Could you check a few things on this model? Use its own coordinates, in mm. A direction names the side the tool comes from. Round coordinates to 2 decimals unless told otherwise and drop trailing zeros. Write each loop counter-clockwise with the first axis right and the second up, starting at its lowest first coordinate (ties: lowest second). Pieces come first, ordered by that corner, then holes. Notation, with made-up numbers: (-2, -39) -> (53, -39) arc R25 ccw to (53, -18) -> close; hole circle Ø2 at (-14, 23.25). An arc over 180 degrees is marked (long way). Answer as CSV lines item,"result". Start each with the question number.
Q1. For faces 1 (the flat face through (34.546, 29, -2)), 2 (the flat face through (26, 31.5, 0)), 3 (the cylindrical face through (22.627, 26.43, -0.488)), 4 (the flat face through (26.946, 0.74, -11.463)), 5 (the flat face through (35, 29, -4.224)), which set-ups out of +Z, -Z, +X, -X, +Y, -Y let a thin tool reach every point of the face, with its end or its side?
Q2. Imagine slicing it at B-B on z = 0.5. Please give me the cut outline in (x, y).
Q3. Imagine slicing it at A-A on y = 28.5. Please give me the cut outline in (x, z), and give its area (3 significant figures).
Q4. Will these pins go through, and if not, where does the flat tip stop? pin 1 Ø2 at (x, z) = (26, -6.5) entering from +Y; pin 2 Ø5 at (x, y) = (20, 5.5) entering from +Z; pin 3 Ø1 at (x, y) = (34.5, 28.5) entering from +Z (3 decimals).
Q5. Imagine slicing it at D-D on y = 12.5. Please give me the cut outline in (x, z), and give its area (3 significant figures).
Q6. If I drill on line 1 (Z direction, x = 26.25, y = 23.5); line 2 (Y direction, x = 33.5, z = 1); line 3 (X direction, y = 19.5, z = 5.75), over which ranges is the centre line in solid material (lowest first)? Write a range as [from, to].
Q7. Imagine slicing it at C-C on x = 25.25. Please give me the cut outline in (y, z), and give its area (3 significant figures).
Q8. If we mould it in two halves opening along Z, with no side actions, what happens to faces 6 (the flat face through (20.605, 28.895, 6.235)), 7 (the flat face through (37.85, 0.74, -0.616)), 8 (the cylindrical face through (30.467, 28.895, 7.089)), 9 (the flat face through (34, 1.5, -7))? For each: pulls with the +Z half, pulls with the -Z half, needs draft (parallel to the pull), parting line crosses it, or undercut.
from build123d import *

# Parameters (mm, degrees)
SKETCH1_R           = 10
SKETCH1_R_2         = 7.636363636
BOSS_EXTRUDE1_DEPTH = 21.5
BOSS_EXTRUDE2_DEPTH = 15
SKETCH3_R           = 3.75
BOSS_EXTRUDE3_DEPTH = 10
BOSS_EXTRUDE4_DEPTH = 1.5
SKETCH6_W           = 32.555421104
SKETCH6_H           = 30.593451785
BOSS_EXTRUDE5_DEPTH = 1.5
SKETCH8_W           = 32.555421103
SKETCH8_H           = 30.593451785
CUT_EXTRUDE1_DEPTH  = 1.5


# Read off the part's stored shape, not the designer's step: Boss-Extrude4
with BuildPart() as part:
    # Sketch1 → Boss-Extrude1 (new body)
    # profile 1 of 2: a face of its own
    with BuildSketch(Plane(origin=(0, 0, 0), x_dir=(1, 0, 0), z_dir=(0, 1, 0))):
        with Locations(Location((0, 0, 0), (0, 0, 270))):
            Circle(SKETCH1_R)
        Circle(SKETCH1_R_2, mode=Mode.SUBTRACT)
    # profile 2 of 2: a face of its own
    with BuildSketch(Plane(origin=(0, 0, 0), x_dir=(1, 0, 0), z_dir=(0, 1, 0))):
        Circle(SKETCH1_R_2)
    extrude(amount=BOSS_EXTRUDE1_DEPTH)

    # Sketch2 → Boss-Extrude2 (add)
    with BuildSketch(Plane(origin=(0, 21.5, 0), x_dir=(1, 0, 0), z_dir=(0, 1, 0))):
        with BuildLine():
            ThreePointArc((3.849666815, -7.240170261), (-4.223312214, -7.028771866), (-8.2, 0))
            Line((-8.2, 0), (-10, 0))
            ThreePointArc((-10, 0), (-5.150380749, -8.571673007), (4.694715628, -8.829475929))
            Line((4.694715628, -8.829475929), (3.849666815, -7.240170261))
        make_face()
        with BuildLine():
            Line((7.578915355, -5.257293639), (3.849666815, -7.240170261))
            Line((3.849666815, -7.240170261), (4.694715628, -8.829475929))
            ThreePointArc((4.694715628, -8.829475929), (6.493411832, -7.604972241), (7.984663341, -6.020394615))
            Line((7.984663341, -6.020394615), (7.578915355, -5.257293639))
        make_face()
        with BuildLine():
            Line((-10, 0), (-8.2, 0))
            Line((-8.2, 0), (-8.2, 4.223635209))
            Line((-8.2, 4.223635209), (-9.064265311, 4.223635209))
            ThreePointArc((-9.064265311, 4.223635209), (-9.763264134, 2.163024144), (-10, 0))
        make_face()
    extrude(amount=BOSS_EXTRUDE2_DEPTH)

    # Sketch3 → Boss-Extrude3 (add)
    with BuildSketch(Plane(origin=(0, 21.5, 0), x_dir=(1, 0, 0), z_dir=(0, 1, 0))):
        with Locations(Location((0, 0, 0), (0, 0, 270))):
            Circle(SKETCH3_R)
    extrude(amount=BOSS_EXTRUDE3_DEPTH)

    # Boss-Extrude4 outline → Boss-Extrude4 (add)
    with BuildSketch(Plane(origin=(0, 0, 0), x_dir=(1, 0, 0), z_dir=(0, 1, 0))):
        with BuildLine():
            ThreePointArc((-0.680367431, 12.982183952), (-9.183045771, 9.201721054), (-12.980774925, 0.706740657))
            Line((-12.980774925, 0.706740657), (-9.986295348, 0.523359562))
            Line((-9.986295348, 0.523359562), (-1.440215285, 0))
            Line((-1.440215285, 0), (0, 0))
            Line((0, 0), (-0.523359562, 9.986295348))
            Line((-0.523359562, 9.986295348), (-0.680367431, 12.982183952))
        make_face()
    extrude(amount=BOSS_EXTRUDE4_DEPTH)

    # Sketch6 → Boss-Extrude5 (add)
    with BuildSketch(Plane.XZ):
        with Locations((-3.104949277, 0.730287835)):
            Rectangle(SKETCH6_W, SKETCH6_H)
    extrude(amount=BOSS_EXTRUDE5_DEPTH)


with BuildPart() as body_2:
    # Mirror6: mirrored copy
    add(part.part.mirror(Plane(origin=(13.172761275, -1.5, 16.027013728), x_dir=(0, 0, 1), z_dir=(-1, 0, 0))))

    # Sketch8 → Cut-Extrude1 (cut)
    with BuildSketch(Plane.XZ.offset(1.5)):
        with Locations((29.450471826, 0.730287835)):
            Rectangle(SKETCH8_W, SKETCH8_H)
    extrude(amount=-CUT_EXTRUDE1_DEPTH, mode=Mode.SUBTRACT)


solid = body_2.part
Checks:
1,face 1,"-Z, +Y"
1,face 2,"-Z, -X, +Y"
1,face 3,"+Y"
1,face 4,"-Z, -X, +Y, -Y"
1,face 5,"-Z, +X, -X, +Y"
2,outline,"(16.36, 0) -> (36.33, 0) -> (36.33, 36.5) -> (34.53, 36.5) -> (34.53, 21.5) -> (30.06, 21.5) -> (30.06, 31.5) -> (22.63, 31.5) -> (22.63, 21.5) -> (16.36, 21.5) -> close"
3,outline,"(18.36, 6.02) -> (18.77, 5.26) -> (22.5, 7.24) arc R8.2 cw to (34.55, 0) -> (34.55, -4.22) -> (35.41, -4.22) arc R10 ccw to start; circle Ø7.5 at (26.35, 0)"
3,area,"90.5 mm^2"
4,pin 1,"y = 21.5"
4,pin 2,"z = 9.23"
4,pin 3,"z = 6.435"
5,outline,"circle Ø20 at (26.35, 0)"
5,area,"314 mm^2"
6,line 1,"[-3.75, 3.75], [8.2, 10]"
6,line 2,"[0, 21.5]"
6,line 3,"[18.16, 34.53]"
7,outline,"(0, -9.94) -> (21.5, -9.94) -> (21.5, -3.59) -> (31.5, -3.59) -> (31.5, 3.59) -> (21.5, 3.59) -> (21.5, 8.13) -> (36.5, 8.13) -> (36.5, 9.94) -> (0, 9.94) -> close"
7,area,"526 mm^2"
8,face 6,"pulls with the -Z half"
8,face 7,"pulls with the +Z half"
8,face 8,"undercut"
8,face 9,"needs draft"
